```python
from build123d import *

# Parameters (mm, degrees)
SKETCH1_R           = 14.2
BOSS_EXTRUDE1_DEPTH = 59
SKETCH2_R           = 2
BOSS_EXTRUDE2_DEPTH = 17.8
SKETCH3_R           = 1.5
CUT_EXTRUDE1_DEPTH  = 4.3942


with BuildPart() as part:
    # Sketch1 → Boss-Extrude1 (new body)
    with BuildSketch(Plane.XY):
        Circle(SKETCH1_R)
    extrude(amount=BOSS_EXTRUDE1_DEPTH)

    # Sketch2 → Boss-Extrude2 (add)
    with BuildSketch(Plane.XY.offset(59)):
        Circle(SKETCH2_R)
    extrude(amount=BOSS_EXTRUDE2_DEPTH)

    # Sketch3 → Cut-Extrude1 (cut)
    with BuildSketch(Plane.XY.offset(59)):
        with Locations((-8.5, 0)):
            Circle(SKETCH3_R)
        with Locations((8.5, 0)):
            Circle(SKETCH3_R)
    extrude(amount=-CUT_EXTRUDE1_DEPTH, mode=Mode.SUBTRACT)


solid = part.part
```
Design review of the part built by this model. Coordinates are the model's own, in mm. A direction names the side the tool comes from. Give positions to 0.01 mm unless a question says otherwise; leave off trailing zeros. Loops run counter-clockwise (first coordinate to the right, second up) from the corner with the lowest first, then second, coordinate; pieces in that order, holes last. Notation, with made-up numbers: (-4, 28.25) -> (42, 28.25) arc R13 cw to (42, 32.25) -> close; hole circle Ø6 at (53, 89.5). An arc over 180 degrees is marked (long way). One line per item, written item: value.
Q1. We need section D-D on z = 32. Give the boundary of the cut face in (x, y).
Numbers:
outline: circle Ø28.4 at (0, 0)
Q2. We need section C-C on z = 57. Give the boundary of the cut face in (x, y).
Numbers:
outline: circle Ø28.4 at (0, 0); hole circle Ø3 at (-8.5, 0); hole circle Ø3 at (8.5, 0)
Q3. Machinability: for faces 5 (the flat face through (0, 0, 0)), 6 (the flat face through (8, 0, 54.606)), which of the approach directions +Z, -Z, +X, -X, +Y, -Y give a long, thin tool a straight path to every point of the face, cutting with its end or side? Answer none if there is none.
Numbers:
face 5: -Z, +X, -X, +Y, -Y
face 6: +Z
Q4. We need section B-B on y = 0. Give the boundary of the cut face in (x, z).
Numbers:
outline: (-14.2, 0) -> (14.2, 0) -> (14.2, 59) -> (10, 59) -> (10, 54.61) -> (7, 54.61) -> (7, 59) -> (2, 59) -> (2, 76.8) -> (-2, 76.8) -> (-2, 59) -> (-7, 59) -> (-7, 54.61) -> (-10, 54.61) -> (-10, 59) -> (-14.2, 59) -> close
Q5. For pin 1 Ø2.5 at (x, y) = (-8.5, 0) entering from +Z; pin 2 Ø10 at (x, y) = (-4, -10) entering from +Z; pin 3 Ø4 at (y, z) = (3, 45) entering from -X, all flat-tipped, find the tip position at first contact; note any pin that passes through.
Numbers:
pin 1: stops at z = 54.61
pin 2: stops at z = 59
pin 3: stops at x = -14.16
Q6. We need section A-A on x = 0. Give the boundary of the cut face in (y, z), and give its area (3 significant figures).
Numbers:
outline: (-14.2, 0) -> (14.2, 0) -> (14.2, 59) -> (2, 59) -> (2, 76.8) -> (-2, 76.8) -> (-2, 59) -> (-14.2, 59) -> close
area: 1,750 mm^2
Q7. Draft analysis for pull direction X (two halves, no side actions). For faces 1 (the cylindrical face through (7.3, -0.9, 56.8)), 2 (the cylindrical face through (-10, 0, 57)), 3 (the flat face through (3, 0, 59)), 4 (the cylindrical face through (0, -2, 68)), state which applies: pulls with the +X half, pulls with the -X half, needs draft (parallel to the pull), parting line crosses it, or undercut.
Numbers:
face 1: undercut
face 2: undercut
face 3: needs draft
face 4: parting line crosses it
Q8. For L1, parallel to Z at x = -7, y = -12; L2, parallel to Y at x = -8, z = 57; L3, parallel to Y at x = 8.5, z = 55.65, list the stretches that pass through material, from the lowest coordinate up.
Numbers:
L1: z = 0 to 59
L2: y = -11.73 to -1.41, 1.41 to 11.73
L3: y = -11.37 to -1.5, 1.5 to 11.37
